Autodesk Inventor part; units mm, degrees
ref_plane "YZ Plane" through (0, 0, 0) normal (1, 0, 0) x (0, 1, 0)
ref_plane "XZ Plane" through (0, 0, 0) normal (0, 1, 0) x (-1, 0, 0)
ref_plane "XY Plane" through (0, 0, 0) normal (0, 0, 1) x (1, 0, 0)
sketch "Sketch1" plane through (0, 0, 0) normal (0, 0, 1) x (1, 0, 0)
  circle A0 centre (0, 0) radius 7.5
  circle A1 centre (0, 0) radius 8.5
  dimension "d0" = 15
  dimension "d1" = 17
extrude "Extrusion1" add sketch "Sketch1" against normal mid plane 25
sketch "Sketch2" plane through (0, 0, 12.5) normal (0, 0, 1) x (1, 0, 0)
  line L0 (-2.75, 9.35) -> (-2.75, 6.9776)
  arc A0 (-2.25, 9.85) -> (-2.75, 9.35) centre (-2.25, 9.35) ccw
  line L1 (2.25, 9.85) -> (-2.25, 9.85)
  arc A1 (2.75, 9.35) -> (2.25, 9.85) centre (2.25, 9.35) ccw
  line L2 (2.75, 6.9776) -> (2.75, 9.35)
  circle A2 centre (0, 0) radius 8.5
  circle A3 centre (0, 0) radius 7.5
  line L3 (-2.75, 6.9776) -> (2.75, 6.9776)
extrude "Extrusion2" cut sketch "Sketch2" against normal blind 7.5 contours A0 L1 A1 L2 A2 L0 | A2 L2 A3 L0 | A3 L3 picked at (1.6937, 7.9533) picked at (-0.4665, 7.1078)
mirror "Mirror1" about plane through (0, 0, 0) normal (0, 0, 1) of "Extrusion2"
properties part number "Pernament magnet" material "Stainless Steel AISI 304"
Part model, mm, in its own coordinate system. A direction names the side the tool comes from. Round coordinates to 2 decimals unless told otherwise and drop trailing zeros. Loops run counter-clockwise (first coordinate to the right, second up) from the corner with the lowest first, then second, coordinate; pieces in that order, holes last. Notation, with made-up numbers: (34.25, 4) -> (77.25, 4) arc R14 cw to (77.25, 24) -> close; hole circle Ø4 at (63.25, -40). An arc over 180 degrees is marked (long way). Use a Markdown table: item, result.
1) Probe line 1 (X direction, y = 0, z = 3.5); line 2 (X direction, y = 4, z = -3.75); line 3 (Y direction, x = 0, z = -6.5). List the from-to ranges inside material, lowest first. Write a range as [from, to].
The answers:
| item | result |
|---|---|
| line 1 | x = [-8.5, -7.5], [7.5, 8.5] |
| line 2 | x = [-7.5, -6.34], [6.34, 7.5] |
| line 3 | y = [-8.5, -7.5] |
2) Cut at C-C, the plane z = -2.75. List the corners of the cut face in (x, y).
The answers:
| item | result |
|---|---|
| outline | circle Ø17 at (0, 0); hole circle Ø15 at (0, 0) |
3) Pull direction X, two halves, no side cores. Call faces 4 (the cylindrical face through (-1.84, -8.3, 0.18)), 5 (the flat face through (0, 8, 5)), 6 (the flat face through (1, -8, 12.5)): pulls with the +X half, pulls with the -X half, needs draft (parallel to the pull), parting line crosses it, or undercut.
The answers:
| item | result |
|---|---|
| face 4 | parting line crosses it |
| face 5 | undercut |
| face 6 | needs draft |
4) Cut at D-D, the plane z = -7.75. List the corners of the cut face in (x, y).
The answers:
| item | result |
|---|---|
| outline | (-2.75, 6.98) -> (-2.75, 8.04) arc R8.5 ccw (long way) to (2.75, 8.04) -> (2.75, 6.98) arc R7.5 cw (long way) to start |
5) Tool access for faces 1 (the flat face through (2.75, 7.5, 8.8)), 2 (the flat face through (-2.75, 7.5, -8.8)), 3 (the flat face through (1, -8, -12.5)): list every direction of +Z, -Z, +X, -X, +Y, -Y with a clear straight run to the whole face (end or side of a thin tool).
The answers:
| item | result |
|---|---|
| face 1 | +Z, +Y |
| face 2 | -Z, +Y |
| face 3 | -Z, +X, -X, +Y, -Y |
6) Drop flat-ended pins along their axis: pin 1 Ø4 at (x, z) = (6.5, 3) entering from -Y; pin 2 Ø1.2 at (y, z) = (7.5, 7.5) entering from -X; pin 3 Ø0.9 at (y, z) = (7.5, -7.5) entering from +X. Give the stop position or say it passes through.
The answers:
| item | result |
|---|---|
| pin 1 | stops at y = -7.21 |
| pin 2 | stops at x = -4.96 |
| pin 3 | stops at x = 4.75 |
7) Cut at B-B, the plane x = 0. List the corners of the cut face in (y, z).
The answers:
| item | result |
|---|---|
| outline | (-8.5, -12.5) -> (-7.5, -12.5) -> (-7.5, 12.5) -> (-8.5, 12.5) -> close; (7.5, -5) -> (8.5, -5) -> (8.5, 5) -> (7.5, 5) -> close |
8) Cut at A-A, the plane y = 0. List the corners of the cut face in (x, z), and give its area (3 significant figures).
The answers:
| item | result |
|---|---|
| outline | (-8.5, -12.5) -> (-7.5, -12.5) -> (-7.5, 12.5) -> (-8.5, 12.5) -> close; (7.5, -12.5) -> (8.5, -12.5) -> (8.5, 12.5) -> (7.5, 12.5) -> close |
| area | 50.0 mm2 |
